from build123d import *

# Parameters (mm, degrees)
SKETCH1_R                = 10
SKETCH1_R_2              = 7.5
BOSS_EXTRUDE1_DEPTH      = 15
BOSS_EXTRUDE2_DEPTH      = 10
BOSS_EXTRUDE2_DEPTH_BACK = 3
SKETCH3_R                = 25
FILLET1_R                = 2
SKETCH4_R                = 15
CUT_EXTRUDE1_DEPTH       = 8
FILLET2_R                = 5


with BuildPart() as part:
    # Sketch1 → Boss-Extrude1 (new body)
    with BuildSketch(Plane(origin=(0, 0, 0), x_dir=(1, 0, 0), z_dir=(0, 1, 0))):
        with Locations(Location((0, 0, 0), (0, 0, 270))):
            Circle(SKETCH1_R)
        with Locations(Location((0, 0, 0), (0, 0, 270))):
            Circle(SKETCH1_R_2, mode=Mode.SUBTRACT)
    extrude(amount=BOSS_EXTRUDE1_DEPTH)

    # Sketch3 → Boss-Extrude2 (add, two sides: drawn at the far end of the back side and taken through both)
    with BuildSketch(Plane(origin=(0, 15, 0), x_dir=(1, 0, 0), z_dir=(0, 1, 0)).offset(-BOSS_EXTRUDE2_DEPTH_BACK)):
        with Locations(Location((0, 0, 0), (0, 0, 270))):
            Circle(SKETCH3_R)
    extrude(amount=BOSS_EXTRUDE2_DEPTH + BOSS_EXTRUDE2_DEPTH_BACK)

    # Fillet1
    fillet1_edges = [part.edges().sort_by_distance(p)[0] for p in [
        (0, 12, -25),
        (0, 25, -25),
    ]]
    fillet(fillet1_edges, radius=FILLET1_R)

    # Sketch4 → Cut-Extrude1 (cut)
    with BuildSketch(Plane(origin=(0, 25, 0), x_dir=(1, 0, 0), z_dir=(0, 1, 0))):
        with Locations(Location((0, 0, 0), (0, 0, 270))):
            Circle(SKETCH4_R)
    extrude(amount=-CUT_EXTRUDE1_DEPTH, mode=Mode.SUBTRACT)

    # Fillet2
    fillet2_edges = [part.edges().sort_by_distance(p)[0] for p in [
        (0, 25, -15),
    ]]
    fillet(fillet2_edges, radius=FILLET2_R)


solid = part.part
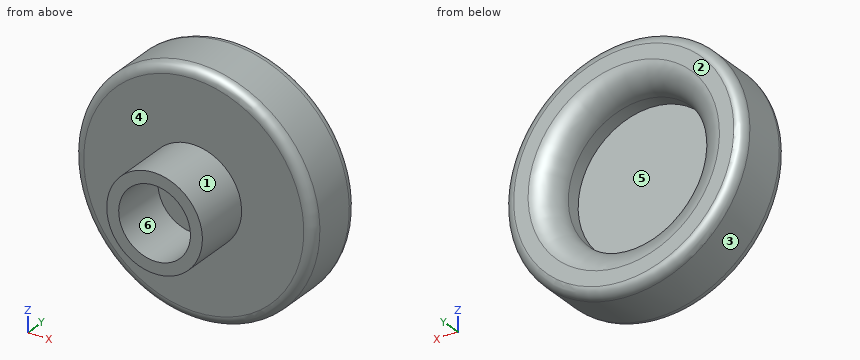
Design review of the part built by this model. Coordinates are the model's own, in mm. Face numbers are marked on the shaded views. A direction names the side the tool comes from. Coordinates: 2 decimals unless noted, no trailing zeros. Write each loop counter-clockwise with the first axis right and the second up, starting at its lowest first coordinate (ties: lowest second). Pieces come first, ordered by that corner, then holes. Notation, with made-up numbers: (32.5, 80) - (43.5, 80) arc R23 cw to (43.5, 113) - close; hole circle Ø6 at (-38.5, 8). An arc over 180 degrees is marked (long way). One line per item, written item: value.
1) Insertion check: pin 1 (4 mm diameter, centred on x = 3, z = -9, fed in from -Y); pin 2 (15 mm diameter, centred on x = -2, z = 0, fed in from +Y); pin 3 (4.5 mm diameter, centred on x = 1.5, z = 3, fed in from -Y); pin 4 (2 mm diameter, centred on y = 12, z = -1, fed in from +X). Each pin has a flat end and moves straight along its axis. Give the tip position at first contact, or say it passes through.
Answer sheet:
pin 1: stops at y = 0
pin 2: stops at y = 17
pin 3: stops at y = 12
pin 4: stops at x = 24.71
2) Add section B-B (x = 0). State the section outline as (y, z) points.
Answer sheet:
outline: (0, -10) - (12, -10) - (12, -23) arc R2 ccw to (14, -25) - (23, -25) arc R2 ccw to (25, -23) - (25, -20) arc R5 ccw to (20, -15) - (17, -15) - (17, 15) - (20, 15) arc R5 ccw to (25, 20) - (25, 23) arc R2 ccw to (23, 25) - (14, 25) arc R2 ccw to (12, 23) - (12, 10) - (0, 10) - (0, 7.5) - (12, 7.5) - (12, -7.5) - (0, -7.5) - close
3) Mouldability with a two-part tool opening along Z and no side actions: class the marked faces 3, 4, 5 and 6 as +Z half, -Z half, draft (parallel to the pull), parting line (faces both ways), or undercut.
Answer sheet:
face 3: parting line
face 4: draft
face 5: undercut
face 6: undercut
4) Add section D-D (y = 17.75). State the section outline as (x, z) points.
Answer sheet:
outline: circle Ø50 at (0, 0); hole circle Ø30 at (0, 0)
5) To check wall thickness, follow probe 1 along Z at (x, y) = (0, 2.5); probe 2 along X at (y, z) = (19.2, 0). State the ranges of each line that lie inside material, in increasing order.
Answer sheet:
probe 1: z = -10 to -7.5, 7.5 to 10
probe 2: x = -25 to -15, 15 to 25
6) Add section C-C (z = 0). State the section outline as (x, y) points.
Answer sheet:
outline: (-25, 14) arc R2 ccw to (-23, 12) - (-10, 12) - (-10, 0) - (-7.5, 0) - (-7.5, 12) - (7.5, 12) - (7.5, 0) - (10, 0) - (10, 12) - (23, 12) arc R2 ccw to (25, 14) - (25, 23) arc R2 ccw to (23, 25) - (20, 25) arc R5 ccw to (15, 20) - (15, 17) - (-15, 17) - (-15, 20) arc R5 ccw to (-20, 25) - (-23, 25) arc R2 ccw to (-25, 23) - close
7) Add section A-A (y = 4.75). State the section outline as (x, z) points, plus the area to 3 significant figures.
Answer sheet:
outline: circle Ø20 at (0, 0); hole circle Ø15 at (0, 0)
area: 137 mm2
8) For the marked faces 1 and 2, list the 3-axis set-ups (+Z, -Z, +X, -X, +Y, -Y) from which the entire face can be reached by the end or side of a thin tool; tool diameter is ignored.
Answer sheet:
face 1: -Y
face 2: +Z, -Z, +X, -X, +Y
